Check sheet for the modelled part. Datum: model origin and axes. Units: mm. A direction names the side the tool comes from. Coordinates: 2 decimals unless noted, no trailing zeros. Loops run counter-clockwise (first coordinate to the right, second up) from the corner with the lowest first, then second, coordinate; pieces in that order, holes last.
```python
from build123d import *

# Parameters (mm, degrees)
SKETCH_1_R             = 7.5
EXTRUDE_1_DEPTH        = 16.5
SKETCH_2_R             = 1.5
EXTRUDE_2_DEPTH        = 10
SKETCH_3_W             = 3.798806197
SKETCH_3_H             = 0.511244187
CUT_EXTRUDE_1_DEPTH    = 7.5
HOLE_WIZARD_M2_1_D     = 1.6
HOLE_WIZARD_M2_1_DEPTH = 6
HOLE_WIZARD_M2_1_TIP   = 0.461880215


with BuildPart() as part:
    # 草图1 → 凸台-拉伸1 (new body)
    with BuildSketch(Plane.XY):
        Circle(SKETCH_1_R)
    extrude(amount=EXTRUDE_1_DEPTH)

    # 草图2 → 凸台-拉伸2 (add)
    with BuildSketch(Plane.XY.offset(16.5)):
        Circle(SKETCH_2_R)
    extrude(amount=EXTRUDE_2_DEPTH)

    # 草图3 → 切除-拉伸1 (cut)
    with BuildSketch(Plane.XY.offset(26.5)):
        with Locations((0.268189439, 1.455622094)):
            Rectangle(SKETCH_3_W, SKETCH_3_H)
    extrude(amount=-CUT_EXTRUDE_1_DEPTH, mode=Mode.SUBTRACT)

    # M2 螺纹孔1
    with Locations(Plane(origin=(5.5, 0, 16.5), x_dir=(1, 0, 0), z_dir=(0, 0, 1))):
        with Locations((0, 0), (-11, 0)):
            Hole(HOLE_WIZARD_M2_1_D / 2, depth=HOLE_WIZARD_M2_1_DEPTH)
            with Locations((0, 0, -(HOLE_WIZARD_M2_1_DEPTH + HOLE_WIZARD_M2_1_TIP / 2))):  # 120° drill point
                Cone(0, HOLE_WIZARD_M2_1_D / 2, HOLE_WIZARD_M2_1_TIP, mode=Mode.SUBTRACT)


solid = part.part
```
1) Mould release check, pull along Y, two halves, no side actions. Record for faces 1 (the flat face through (0, 0, 0)), 2 (the flat face through (0, 1.2, 23)), 3 (the cylindrical face through (-4.7, 0, 13.5)): +Y half, -Y half, draft (parallel to the pull), parting line (faces both ways), or undercut.
Answer sheet:
face 1: draft
face 2: +Y half
face 3: undercut
2) Set-up check for faces 4 (the flat face through (0, 0, 26.5)), 5 (the cylindrical face through (-0.325, -1.464, 21.43)): record each of +Z, -Z, +X, -X, +Y, -Y from which the full face is reachable in a straight line by a thin tool's end or side.
Answer sheet:
face 4: +Z, +X, -X, +Y, -Y
face 5: +Z
3) Section check A-A on z = 20.25. Enter the section's corners in (x, y), plus the area to 3 significant figures.
Answer sheet:
outline: (-0.9, 1.2) arc R1.5 ccw (long way) to (0.9, 1.2) - close
area: 6.70 mm2
4) Scan lines: line 1 (Z direction, x = 1.5, y = -3.5); line 2 (Y direction, x = -5.5, z = 15.05); line 3 (Y direction, x = -4, z = 3). Record each from-to range of solid material in increasing order.
Answer sheet:
line 1: z = 0 to 16.5
line 2: y = -5.1 to -0.8, 0.8 to 5.1
line 3: y = -6.34 to 6.34
5) Section check D-D on x = 4.25. Enter the section's corners in (y, z).
Answer sheet:
outline: (-6.18, 0) - (6.18, 0) - (6.18, 16.5) - (-6.18, 16.5) - close
6) Section check B-B on y = -4.5. Enter the section's corners in (x, z).
Answer sheet:
outline: (-6, 0) - (6, 0) - (6, 16.5) - (-6, 16.5) - close
7) Depth check by flat-ended pin: pin 1 (0.9 mm diameter, centred on x = 0, z = 22.5, fed in from +Y); pin 2 (5 mm diameter, centred on x = 3, y = -3, fed in from +Z); pin 3 (1.5 mm diameter, centred on x = -3, z = 5, fed in from -Y). Enter the tip coordinate at first touch or a pass-through.
Answer sheet:
pin 1: stops at y = 1.2
pin 2: stops at z = 16.5
pin 3: stops at y = -7.15
8) Section check C-C on z = 12.25. Enter the section's corners in (x, y).
Answer sheet:
outline: circle Ø15 at (0, 0); hole circle Ø1.6 at (-5.5, 0); hole circle Ø1.6 at (5.5, 0)
